Check sheet for the modelled part. Datum: model origin and axes. Units: mm. A direction names the side the tool comes from. Round coordinates to 2 decimals unless told otherwise and drop trailing zeros. Order: outer loops, then holes, each group sorted by start corner. A loop starts at its lowest first (then second) coordinate and runs counter-clockwise, first axis right, second up. Notation, with made-up numbers: (89, 60.5) -> (123, 60.5) arc R25 ccw to (123, 79.5) -> close; hole circle Ø9 at (19.5, -25.75). An arc over 180 degrees is marked (long way). Answer in a Markdown table with one row per item.
from build123d import *

# Parameters (mm, degrees)
ESTRUSIONE_ESTRUSIONE1_DEPTH = 50
SMUSSO1_SIZE                 = 1.6
RIVOLUZIONE1_ANGLE           = 14.31
FORO_PER_VITE_M5_2_D         = 5.6
FORO_PER_VITE_M5_2_DEPTH     = 120
FORO_PER_VITE_M5_2_TIP       = 1.682409733


with BuildPart() as part:
    # Schizzo1 → Estrusione-Estrusione1 (new body)
    with BuildSketch(Plane(origin=(0, 0, 0), x_dir=(0, 0, -1), z_dir=(1, 0, 0))):
        with BuildLine():
            Line((-10, -23.5), (-10, -20.5))
            Line((-10, -20.5), (-22.5, -20.5))
            Line((-22.5, -20.5), (-22.5, -9))
            Line((-22.5, -9), (22.5, -9))
            Line((22.5, -9), (22.5, -20.5))
            Line((22.5, -20.5), (10, -20.5))
            Line((10, -20.5), (10, -23.5))
            Line((10, -23.5), (25, -23.5))
            Line((25, -23.5), (25, -2.5))
            Line((25, -2.5), (22.5, -2.5))
            Line((22.5, -2.5), (22.5, -7))
            Line((22.5, -7), (12.5, -7))
            Line((12.5, -7), (12.5, 7))
            Line((12.5, 7), (22.5, 7))
            Line((22.5, 7), (22.5, 2.5))
            Line((22.5, 2.5), (25, 2.5))
            Line((25, 2.5), (25, 19.5))
            ThreePointArc((25, 19.5), (25.585786438, 20.914213562), (27, 21.5))
            Line((27, 21.5), (33, 21.5))
            ThreePointArc((33, 21.5), (35.828427125, 22.671572875), (37, 25.5))
            Line((37, 25.5), (37, 47.5))
            Line((37, 47.5), (35, 47.5))
            Line((35, 47.5), (35, 25.5))
            ThreePointArc((35, 25.5), (34.414213562, 24.085786438), (33, 23.5))
            Line((33, 23.5), (10, 23.5))
            Line((10, 23.5), (10, 20.5))
            Line((10, 20.5), (22.5, 20.5))
            Line((22.5, 20.5), (22.5, 9))
            Line((22.5, 9), (-22.5, 9))
            Line((-22.5, 9), (-22.5, 20.5))
            Line((-22.5, 20.5), (-10, 20.5))
            Line((-10, 20.5), (-10, 23.5))
            Line((-10, 23.5), (-33, 23.5))
            ThreePointArc((-33, 23.5), (-34.414213562, 24.085786438), (-35, 25.5))
            Line((-35, 25.5), (-35, 47.5))
            Line((-35, 47.5), (-37, 47.5))
            Line((-37, 47.5), (-37, 25.5))
            ThreePointArc((-37, 25.5), (-35.828427125, 22.671572875), (-33, 21.5))
            Line((-33, 21.5), (-27, 21.5))
            ThreePointArc((-27, 21.5), (-25.585786438, 20.914213562), (-25, 19.5))
            Line((-25, 19.5), (-25, 2.5))
            Line((-25, 2.5), (-22.5, 2.5))
            Line((-22.5, 2.5), (-22.5, 7))
            Line((-22.5, 7), (-12.5, 7))
            Line((-12.5, 7), (-12.5, -7))
            Line((-12.5, -7), (-22.5, -7))
            Line((-22.5, -7), (-22.5, -2.5))
            Line((-22.5, -2.5), (-25, -2.5))
            Line((-25, -2.5), (-25, -23.5))
            Line((-25, -23.5), (-10, -23.5))
        make_face()
        with BuildLine():
            Line((-8.5, 7), (8.5, 7))
            ThreePointArc((8.5, 7), (9.560660172, 6.560660172), (10, 5.5))
            Line((10, 5.5), (10, -5.5))
            ThreePointArc((10, -5.5), (9.560660172, -6.560660172), (8.5, -7))
            Line((8.5, -7), (-8.5, -7))
            ThreePointArc((-8.5, -7), (-9.560660172, -6.560660172), (-10, -5.5))
            Line((-10, -5.5), (-10, 5.5))
            ThreePointArc((-10, 5.5), (-9.560660172, 6.560660172), (-8.5, 7))
        make_face(mode=Mode.SUBTRACT)
    extrude(amount=ESTRUSIONE_ESTRUSIONE1_DEPTH)

    # Smusso1
    smusso1_edges = [part.edges().sort_by_distance(p)[0] for p in [
        (25, -7, 22.5),
        (25, -7, 12.5),
        (25, 7, 12.5),
        (25, 7, 22.5),
        (25, 7, -22.5),
        (25, 7, -12.5),
        (25, -7, -12.5),
        (25, -7, -22.5),
    ]]
    chamfer(smusso1_edges, length=SMUSSO1_SIZE)

    # Schizzo2 → Rivoluzione1 (revolve)
    with BuildSketch(Plane(origin=(50, 0, 0), x_dir=(0, 0, -1), z_dir=(1, 0, 0))):
        with BuildLine():
            Line((-10, -23.5), (-25, -23.5))
            Line((-25, -23.5), (-25, 19.5))
            ThreePointArc((-25, 19.5), (-25.585786438, 20.914213562), (-27, 21.5))
            Line((-27, 21.5), (-33, 21.5))
            ThreePointArc((-33, 21.5), (-35.828427125, 22.671572875), (-37, 25.5))
            Line((-37, 25.5), (-37, 47.5))
            Line((-37, 47.5), (-35, 47.5))
            Line((-35, 47.5), (-35, 25.5))
            ThreePointArc((-35, 25.5), (-34.414213562, 24.085786438), (-33, 23.5))
            Line((-33, 23.5), (-10, 23.5))
            Line((-10, 23.5), (-10, 20.5))
            Line((-10, 20.5), (-22.5, 20.5))
            Line((-22.5, 20.5), (-22.5, 9))
            Line((-22.5, 9), (22.5, 9))
            Line((22.5, 9), (22.5, 20.5))
            Line((22.5, 20.5), (10, 20.5))
            Line((10, 20.5), (10, 23.5))
            Line((10, 23.5), (33, 23.5))
            ThreePointArc((33, 23.5), (34.414213562, 24.085786438), (35, 25.5))
            Line((35, 25.5), (35, 47.5))
            Line((35, 47.5), (37, 47.5))
            Line((37, 47.5), (37, 25.5))
            ThreePointArc((37, 25.5), (35.828427125, 22.671572875), (33, 21.5))
            Line((33, 21.5), (27, 21.5))
            ThreePointArc((27, 21.5), (25.585786438, 20.914213562), (25, 19.5))
            Line((25, 19.5), (25, -23.5))
            Line((25, -23.5), (10, -23.5))
            Line((10, -23.5), (10, -20.5))
            Line((10, -20.5), (22.5, -20.5))
            Line((22.5, -20.5), (22.5, -9))
            Line((22.5, -9), (-22.5, -9))
            Line((-22.5, -9), (-22.5, -20.5))
            Line((-22.5, -20.5), (-10, -20.5))
            Line((-10, -20.5), (-10, -23.5))
        make_face()
    revolve(axis=Axis((50, 450, 89.886149412), (0, 0, 1)), revolution_arc=RIVOLUZIONE1_ANGLE)

    # Schizzo18 → Taglia-Rivoluzione1 (revolve, cut)
    with BuildSketch(Plane(origin=(154.720013769, 39.4663965, 0), x_dir=(0, 0, -1), z_dir=(0.9689726071879229, 0.24716813411004152, 0))):
        Polygon((-25, -26.320733471), (25, -26.320733471), (25, -21.320733471), (23.5, -21.320733471), (23.5, -23.520733471), (-23.5, -23.520733471), (-23.5, -21.320733471), (-25, -21.320733471), align=None)
    revolve(axis=Axis((161.22566035, 13.962326765, 25), (0, 0, -1)), mode=Mode.SUBTRACT)

    # Foro per Vite M5-2
    with Locations(Plane(origin=(-8.832087888, 0, 67.086367898), x_dir=(0.9914448613738102, 0, 0.13052619222005385), z_dir=(-0.13052619222005385, 0, 0.9914448613738102))):
        with Locations((140.267423642, 11.500002666)):
            Hole(FORO_PER_VITE_M5_2_D / 2, depth=FORO_PER_VITE_M5_2_DEPTH)
            with Locations((0, 0, -(FORO_PER_VITE_M5_2_DEPTH + FORO_PER_VITE_M5_2_TIP / 2))):  # 118° drill point
                Cone(0, FORO_PER_VITE_M5_2_D / 2, FORO_PER_VITE_M5_2_TIP, mode=Mode.SUBTRACT)


solid = part.part
Item 1: Mould release check, pull along X, two halves, no side actions. Record for faces 1 (the cylindrical face through (102.38, 26.73, 21.34)), 2 (the cylindrical face through (102.75, 23.75, -16.16)), 3 (the flat face through (84, -21, 10)), 4 (the flat face through (84, -11, 22.5)): pulls with the +X half, pulls with the -X half, needs draft (parallel to the pull), parting line crosses it, or undercut.
Result sheet:
| item | result |
|---|---|
| face 1 | pulls with the -X half |
| face 2 | undercut |
| face 3 | needs draft |
| face 4 | undercut |
Item 2: Cross-section at B-B (y = 44). Record the boundary of the cut face in (x, z), and give its area (3 significant figures).
Result sheet:
| item | result |
|---|---|
| outline | (0, -37) -> (153.56, -37) -> (153.56, -35) -> (0, -35) -> close; (0, 35) -> (153.56, 35) -> (153.56, 37) -> (0, 37) -> close |
| area | 614 mm^2 |
Item 3: Scan lines: line 1 (Y direction, x = 14.5, z = 15); line 2 (Y direction, x = 23, z = -11.5); line 3 (Y direction, x = 67.5, z = -22). Record each from-to range of solid material in increasing order. Write a range as [from, to].
Result sheet:
| item | result |
|---|---|
| line 1 | y = [-23.5, -20.5], [-9, -7], [7, 9], [20.5, 23.5] |
| line 2 | y = [-23.5, -20.5], [-9, 9], [20.5, 23.5] |
| line 3 | y = [-23.18, -20.17], [-8.67, 9.35], [20.86, 23.86] |
Item 4: Set-up check for faces 5 (the flat face through (25, 21.5, -30)), 6 (the flat face through (25, 20.5, 16)), 7 (the flat face through (25, 23.5, -22)): record each of +Z, -Z, +X, -X, +Y, -Y from which the full face is reachable in a straight line by a thin tool's end or side.
Result sheet:
| item | result |
|---|---|
| face 5 | -Z, +X, -X, -Y |
| face 6 | -X |
| face 7 | -X, +Y |
Item 5: Cross-section at A-A (y = 54.5). Record the boundary of the cut face in (x, z), and give its area (3 significant figures).
Result sheet:
| item | result |
|---|---|
| outline | (124.74, -37) -> (150.89, -37) -> (150.89, -35) -> (124.74, -35) -> close; (124.74, 35) -> (150.89, 35) -> (150.89, 37) -> (124.74, 37) -> close |
| area | 105 mm^2 |
Item 6: Depth check by flat-ended pin: P1, Ø8.5, axis at x = 21, z = 2.5, coming from the +Y side; P2, Ø8.5, axis at x = 16, z = -2, coming from the -Y side; P3, Ø22.5, axis at x = 32, z = -3, coming from the +Y side. Enter the tip coordinate at first touch or a pass-through.
Result sheet:
| item | result |
|---|---|
| P1 | stops at y = 9 |
| P2 | stops at y = -9 |
| P3 | stops at y = 23.5 |
